Autodesk Inventor part; units mm, degrees
ref_plane "YZ Plane" through (0, 0, 0) normal (1, 0, 0) x (0, 1, 0)
ref_plane "XZ Plane" through (0, 0, 0) normal (0, 1, 0) x (-1, 0, 0)
ref_plane "XY Plane" through (0, 0, 0) normal (0, 0, 1) x (1, 0, 0)
sketch "Sketch1" plane through (0, 0, 0) normal (1, 0, 0) x (0, 1, 0)
  line L0 (-228.6, 234.95) -> (228.6, 234.95)
  line L1 (228.6, 234.95) -> (228.6, -234.95)
  line L2 (228.6, -234.95) -> (-228.6, -234.95)
  line L3 (-228.6, -234.95) -> (-228.6, 234.95)
  line L4 (-228.6, 234.95) -> (228.6, -234.95) construction
  line L5 (228.6, 234.95) -> (-228.6, -234.95) construction
  point P0 (0, 0)
  dimension "d0" = 457.2
  dimension "d1" = 469.9
extrude "Extrusion1" add sketch "Sketch1" along normal blind 19.05
sketch "Sketch2" plane through (19.05, 0, 0) normal (1, 0, 0) x (0, 0, -1)
  circle A0 centre (184.15, 0) radius 25.4
  line L0 (234.95, -228.6) -> (234.95, 228.6)
  point P0 (0, 0)
  point P1 (234.95, 0)
  dimension "d4" = 50.8
  dimension "d5" = 50.8
extrude "Extrusion2" add sketch "Sketch2" along normal blind 19.05
sketch "Sketch3" plane through (38.1, 0, -184.15) normal (1, 0, 0) x (0, 0, -1)
  circle A0 centre (0, 0) radius 50.8
  line L0 (50.8, -228.6) -> (50.8, 228.6)
  point P0 (-184.15, 0)
  dimension "d8" = 50.8
  dimension "d9" = 101.6
extrude "Extrusion3" add sketch "Sketch3" along normal blind 50.8
fillet "Fillet1" radius 25.4 2 edges at (88.9, 0, -133.35) (38.1, 0, -133.35)
properties part number "front door (for assembly)"
Geometry: final body of the model. Coordinates: model frame, mm. Round coordinates to 2 decimals unless told otherwise and drop trailing zeros. Order: outer loops, then holes, each group sorted by start corner. A loop starts at its lowest first (then second) coordinate and runs counter-clockwise, first axis right, second up. Notation, with made-up numbers: (58, 88) - (85, 88) arc R25 ccw to (85, 125) - close; hole circle Ø7 at (-7, 67.5). An arc over 180 degrees is marked (long way). Use CSV: the item, a comma, the result in double quotes. Start each with the question number.
Q1. Section query C-C (z = -72). Return loops of the section in (x, y), and give its area (3 significant figures).
Q2. Mould query, pull axis X, two halves, no side actions, for faces 1 (the face through (28.442, -1.117, -158.775)), 2 (the face through (88.9, 0, -184)), 3 (the face through (0, -3, 3)). Classes: +X half, -X half, draft (parallel to the pull), parting line (faces both ways), or undercut.
Q3. Material intervals for line 1 along X through (y, z) = (-207.5, -91); line 2 along Y through (x, z) = (22, -198); line 3 along Y through (x, z) = (79, -178), sorted ascending. Write a range as from..to.
Q4. Section query D-D (x = 52). Return loops of the section in (y, z), and give its area (3 significant figures).
Q5. First-contact query: pin 1 (2 mm diameter, centred on y = 24.5, z = -103, fed in from +X); pin 2 (10 mm diameter, centred on y = -34.5, z = -167.5, fed in from +X). Flat tips, straight axial feed; report the tip coordinate or a pass-through.
Result set:
1,outline,"(0, -228.6) - (19.05, -228.6) - (19.05, 228.6) - (0, 228.6) - close"
1,area,"8,710 mm2"
2,face 1,"undercut"
2,face 2,"+X half"
2,face 3,"-X half"
3,line 1,"x = 0..19.05"
3,line 2,"y = -21.29..21.29"
3,line 3,"y = -45.11..45.11"
4,outline,"circle Ø96.1 at (0, -184.15)"
4,area,"7,250 mm2"
5,pin 1,"stops at x = 19.05"
5,pin 2,"stops at x = 87.64"
